Part print with two shaded views. Sizes in mm from the minimum x, y, z corner. Give positions to 0.01 mm unless a question says otherwise; leave off trailing zeros. Order: outer loops, then holes, each group sorted by start corner. A loop starts at its lowest first (then second) coordinate and runs counter-clockwise, first axis right, second up. Notation, with made-up numbers: M -22,20 L 34,20 A20 cw 34,57 Z; hole C 87.5,53.5 d1. An arc over 180 degrees is marked long. Return JSON: item names as keys, results as strings. Group by question number.
1. Slice it at B-B on x = 21.5. List the corners of the cut face in (y, z).
2. Slice it at C-C on z = 273. List the corners of the cut face in (x, y).
3. Wall check: probe 1 along Z at (x, y) = (16.5, 1.65); probe 2 along X at (y, z) = (1.15, 302.26); probe 3 along Z at (x, y) = (14.5, 2.9) (1 decimal). Give the ranges that are in metal, low to high. Write a range as [from, to].
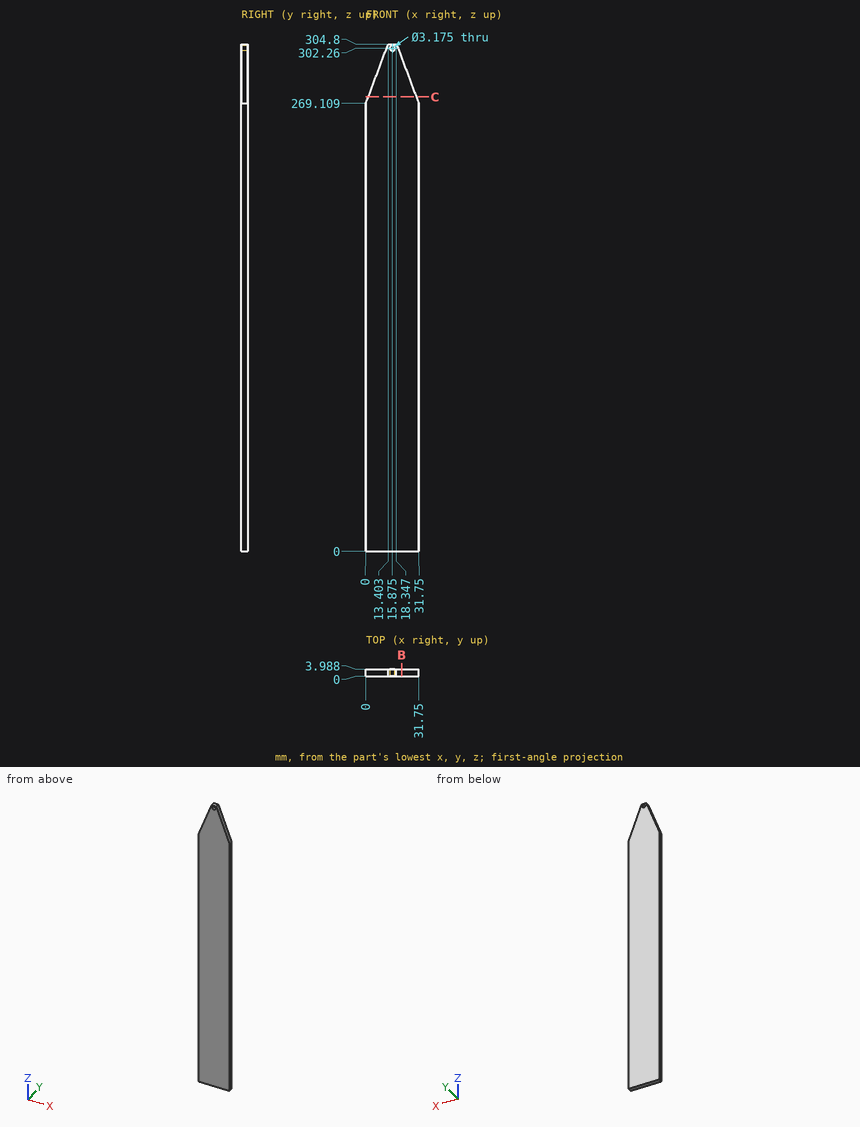
Result:
{
 "1": {"outline": "M 0,0 L 3.99,0 L 3.99,296.4 L 0,296.4 Z"},
 "2": {"outline": "M 1.46,0 L 30.29,0 L 30.29,3.99 L 1.46,3.99 Z"},
 "3": {"probe 1": "z = [0, 300.8], [303.72, 304.8]", "probe 2": "x = [12.45, 14.29], [17.46, 19.3]", "probe 3": "z = [0, 301.5], [303.1, 304.8]"}
}
